Model file for the job. Use its own axes, mm. A direction names the side the tool comes from. Round coordinates to 2 decimals unless told otherwise and drop trailing zeros. Order: outer loops, then holes, each group sorted by start corner. A loop starts at its lowest first (then second) coordinate and runs counter-clockwise, first axis right, second up. Notation, with made-up numbers: (44, -40) - (54, -40) arc R21 ccw to (54, -21) - close; hole circle Ø4 at (76.25, 41). An arc over 180 degrees is marked (long way). Put each result on its own line as item: value. Start each with the question number.
Item 1: Saw through at B-B on z = 55. List the corners of the cut face in (x, y).
Item 2: Saw through at A-A on z = 45. List the corners of the cut face in (x, y).
Item 3: Saw through at D-D on x = 60. List the corners of the cut face in (y, z), plus the area to 3 significant figures.
Item 4: Saw through at C-C on y = 21.25. State how many separate pieces and enclosed holes the cut face has, plus the area to 3 significant figures.
Item 5: Which spindle directions (+Z, -Z, +X, -X, +Y, -Y) get a long thin tool onto all of the face, cutting with end or side? Do faces 3 (the face through (12.6, 31, 70)), 4 (the face through (12, 33, 52)), 5 (the face through (118.084, 34.365, 53.216)). Say none if no direction does.
Item 6: Mould opens along Y. For faces 1 (the face through (118.084, 34.365, 37.216)), 2 (the face through (17.969, 5.407, 53.137)) say: pulls with the +Y half, pulls with the -Y half, needs draft (parallel to the pull), parting line crosses it, or undercut.
Item 7: Pin check, flat tips, straight feed: pin 1 Ø8 at (x, y) = (57.5, 16) entering from -Z; pin 2 Ø1 at (y, z) = (9, 19.5) entering from +X; pin 3 Ø4 at (x, y) = (75, 21.25) entering from +Z. Stop position of each tip, or through.
Item 8: Probe probe 1 along X at (y, z) = (21, 23.5); probe 2 along Z at (x, y) = (17, 7); probe 3 along X at (y, z) = (8.5, 15). List the from-to ranges inside material, lowest first.
```python
from build123d import *

# Parameters (mm, degrees)
SKETCH1_W           = 124
SKETCH1_H           = 42.5
SKETCH1_R           = 10.5
SKETCH1_R_2         = 10
SKETCH1_R_3         = 1.65
BOSS_EXTRUDE1_DEPTH = 70
SKETCH2_W           = 58
SKETCH2_H           = 42.5
CUT_EXTRUDE1_DEPTH  = 46
SKETCH3_R           = 18.35
CUT_EXTRUDE2_DEPTH  = 5
SKETCH5_R           = 1.65
CUT_EXTRUDE4_DEPTH  = 12
SKETCH6_R           = 1.65
CUT_EXTRUDE5_DEPTH  = 12
CUT_EXTRUDE3_REACH  = 44.5
SKETCH4_R           = 2.1


with BuildPart() as part:
    # Sketch1 → Boss-Extrude1 (new body)
    with BuildSketch(Plane.XY):
        with Locations((62, 21.25)):
            Rectangle(SKETCH1_W, SKETCH1_H)
        with Locations((17, 21.25)):
            Circle(SKETCH1_R, mode=Mode.SUBTRACT)
        with Locations((62, 21.25)):
            Circle(SKETCH1_R_2, mode=Mode.SUBTRACT)
        with Locations((107, 21.25)):
            Circle(SKETCH1_R, mode=Mode.SUBTRACT)
        with Locations((49, 21.25)):
            Circle(SKETCH1_R_3, mode=Mode.SUBTRACT)
        with Locations((75, 21.25)):
            Circle(SKETCH1_R_3, mode=Mode.SUBTRACT)
    extrude(amount=BOSS_EXTRUDE1_DEPTH)

    # Sketch2 → Cut-Extrude1 (cut)
    with BuildSketch(Plane.XY.offset(70)):
        with Locations((62, 21.25)):
            Rectangle(SKETCH2_W, SKETCH2_H)
    extrude(amount=-CUT_EXTRUDE1_DEPTH, mode=Mode.SUBTRACT)

    # Sketch3 → Cut-Extrude2 (cut)
    with BuildSketch(Plane(origin=(0, 0, 0), x_dir=(-1, 0, 0), z_dir=(0, 0, -1))):
        with Locations((-62, 21.25)):
            Circle(SKETCH3_R)
    extrude(amount=-CUT_EXTRUDE2_DEPTH, mode=Mode.SUBTRACT)

    # Sketch5 → Cut-Extrude4 (cut)
    with BuildSketch(Plane(origin=(124, 0, 0), x_dir=(0, 0, -1), z_dir=(1, 0, 0))):
        with Locations((-20, 9.25)):
            Circle(SKETCH5_R)
        with Locations((-20, 33.25)):
            Circle(SKETCH5_R)
        with Locations((-36, 33.25)):
            Circle(SKETCH5_R)
        with Locations((-36, 9.25)):
            Circle(SKETCH5_R)
        with Locations((-52, 9.25)):
            Circle(SKETCH5_R)
        with Locations((-52, 33.25)):
            Circle(SKETCH5_R)
        with Locations((-66, 21.25)):
            Circle(SKETCH5_R)
        with Locations((-4, 21.25)):
            Circle(SKETCH5_R)
    extrude(amount=-CUT_EXTRUDE4_DEPTH, mode=Mode.SUBTRACT)

    # Sketch6 → Cut-Extrude5 (cut)
    with BuildSketch(Plane.ZY):
        with Locations((20, 33.25)):
            Circle(SKETCH6_R)
        with Locations((36, 33.25)):
            Circle(SKETCH6_R)
        with Locations((36, 9.25)):
            Circle(SKETCH6_R)
        with Locations((20, 9.25)):
            Circle(SKETCH6_R)
        with Locations((52, 33.25)):
            Circle(SKETCH6_R)
        with Locations((52, 9.25)):
            Circle(SKETCH6_R)
        with Locations((66, 21.25)):
            Circle(SKETCH6_R)
        with Locations((4, 21.25)):
            Circle(SKETCH6_R)
    extrude(amount=-CUT_EXTRUDE5_DEPTH, mode=Mode.SUBTRACT)

    # Sketch4 → Cut-Extrude3 (cut, up to next)
    with BuildSketch(Plane.XZ, mode=Mode.PRIVATE) as cut_extrude3_sk1:
        with Locations((17, 55)):
            Circle(SKETCH4_R)
    cut_extrude3_tool1 = extrude(cut_extrude3_sk1.sketch, amount=-CUT_EXTRUDE3_REACH, mode=Mode.PRIVATE) & part.part
    add(cut_extrude3_tool1.solids().sort_by_distance((17, 0, 55))[0], mode=Mode.SUBTRACT)
    # Sketch4 → Cut-Extrude3 (cut, up to next)
    with BuildSketch(Plane.XZ, mode=Mode.PRIVATE) as cut_extrude3_sk2:
        with Locations((17, 15)):
            Circle(SKETCH4_R)
    cut_extrude3_tool2 = extrude(cut_extrude3_sk2.sketch, amount=-CUT_EXTRUDE3_REACH, mode=Mode.PRIVATE) & part.part
    add(cut_extrude3_tool2.solids().sort_by_distance((17, 0, 15))[0], mode=Mode.SUBTRACT)
    # Sketch4 → Cut-Extrude3 (cut, up to next)
    with BuildSketch(Plane.XZ, mode=Mode.PRIVATE) as cut_extrude3_sk3:
        with Locations((107, 15)):
            Circle(SKETCH4_R)
    cut_extrude3_tool3 = extrude(cut_extrude3_sk3.sketch, amount=-CUT_EXTRUDE3_REACH, mode=Mode.PRIVATE) & part.part
    add(cut_extrude3_tool3.solids().sort_by_distance((107, 0, 15))[0], mode=Mode.SUBTRACT)
    # Sketch4 → Cut-Extrude3 (cut, up to next)
    with BuildSketch(Plane.XZ, mode=Mode.PRIVATE) as cut_extrude3_sk4:
        with Locations((107, 55)):
            Circle(SKETCH4_R)
    cut_extrude3_tool4 = extrude(cut_extrude3_sk4.sketch, amount=-CUT_EXTRUDE3_REACH, mode=Mode.PRIVATE) & part.part
    add(cut_extrude3_tool4.solids().sort_by_distance((107, 0, 55))[0], mode=Mode.SUBTRACT)


solid = part.part
```
Results found:
1. outline: (0, 0) - (14.9, 0) - (14.9, 10.96) arc R10.5 cw (long way) to (19.1, 10.96) - (19.1, 0) - (33, 0) - (33, 42.5) - (0, 42.5) - close; (91, 0) - (104.9, 0) - (104.9, 10.96) arc R10.5 cw (long way) to (109.1, 10.96) - (109.1, 0) - (124, 0) - (124, 42.5) - (91, 42.5) - close
2. outline: (0, 0) - (33, 0) - (33, 42.5) - (0, 42.5) - close; (91, 0) - (124, 0) - (124, 42.5) - (91, 42.5) - close; hole circle Ø21 at (17, 21.25); hole circle Ø21 at (107, 21.25)
3. outline: (0, 0) - (3.01, 0) - (3.01, 5) - (11.45, 5) - (11.45, 24) - (0, 24) - close; (31.05, 5) - (39.49, 5) - (39.49, 0) - (42.5, 0) - (42.5, 24) - (31.05, 24) - close
3. area: 465 mm²
4. separate pieces: 10
4. enclosed holes: 0
4. area: 2,300 mm²
5. face 3: +Z, +X, -X, +Y, -Y
5. face 4: -X
5. face 5: +X
6. face 1: undercut
6. face 2: needs draft
7. pin 1: stops at z = 5
7. pin 2: stops at x = 112
7. pin 3: stops at z = 24
8. probe 1: x = 0 to 6.5, 27.5 to 47.37, 50.63 to 52, 72 to 73.37, 76.63 to 96.5, 117.5 to 124
8. probe 2: z = 0 to 12.9, 17.1 to 52.9, 57.1 to 70
8. probe 3: x = 0 to 14.9, 19.1 to 104.9, 109.1 to 124
